Here's how the part is built. I have some questions about the finished solid (model axes, mm). Give positions to 0.01 mm unless a question says otherwise; leave off trailing zeros. Loops run counter-clockwise (first coordinate to the right, second up) from the corner with the lowest first, then second, coordinate; pieces in that order, holes last. Notation, with made-up numbers: (36, 66.5) - (46, 66.5) arc R24 cw to (46, 99.5) - close; hole circle Ø5 at (72.25, 60). An arc over 180 degrees is marked (long way). Use one line per item in the form item = value.
from build123d import *

# Parameters (mm, degrees)
F0_W     = 19.05
F0_H     = 19.05
F0_W_2   = 12.7
F1_DEPTH = 7.9375
F2_D     = 10.0838
F3_D     = 13.49248


# Not quite as in the source:
# - a feature names something its author has since deleted; it is built from what else it names


with BuildPart() as f1:
    # F0 (on Top) → F1 (new body)
    with BuildSketch(Plane.XY):
        with Locations((-66.5298237595, -51.1898304701)):
            Rectangle(F0_W, F0_H)
        Polygon((-57.0048237595, -41.6648304701), (-57.0048237595, -60.7148304701), (-37.9548237595, -60.7148304701), (-37.9548237595, 9.1351695299), (-76.0548237595, 9.1351695299), (-76.0548237595, -41.6648304701), align=None)
        Polygon((-37.9548237595, 9.1351695299), (-37.9548237595, -60.7148304701), (0.1451762405, -60.7148304701), (0.1451762405, -41.6648304701), (0.1451762405, -0.3898304701), (22.3701762405, -0.3898304701), (22.3701762405, -41.6648304701), (22.3701762405, -60.7148304701), (38.2451762405, -60.7148304701), (38.2451762405, 9.1351695299), align=None)
        Polygon((-37.9548237595, 78.9851695299), (-76.0548237595, 9.1351695299), (-37.9548237595, 9.1351695299), (-37.9548237595, 59.9351695299), align=None)
        Polygon((0.1451762405, -41.6648304701), (0.1451762405, -60.7148304701), (22.3701762405, -60.7148304701), (22.3701762405, -41.6648304701), (22.3701762405, -0.3898304701), (0.1451762405, -0.3898304701), align=None)
        Polygon((-37.9548237595, 59.9351695299), (-37.9548237595, 9.1351695299), (38.2451762405, 9.1351695299), (38.2451762405, 59.9351695299), (25.5451762405, 59.9351695299), (25.5451762405, 78.9851695299), (-25.2548237595, 78.9851695299), (-25.2548237595, 59.9351695299), align=None)
        with Locations((-31.6048237595, 69.4601695299)):
            Rectangle(F0_W_2, F0_H)
        Polygon((38.2451762405, 59.9351695299), (38.2451762405, 9.1351695299), (76.3451762405, 9.1351695299), (38.2451762405, 78.9851695299), align=None)
        Polygon((76.3451762405, 9.1351695299), (38.2451762405, 9.1351695299), (38.2451762405, -60.7148304701), (57.2951762405, -60.7148304701), (76.3451762405, -60.7148304701), align=None)
        with Locations((31.8951762405, 69.4601695299)):
            Rectangle(F0_W_2, F0_H)
    extrude(amount=F1_DEPTH)

    # F2 (through all)
    with Locations(Plane(origin=(0, 0, 0), x_dir=(1, 0, 0), z_dir=(0, 0, -1))):
        with Locations((-57.0048237595, 0.3898304701), (-57.0048237595, 41.6648304701), (0.1451762405, 0.3898304701), (0.1451762405, 41.6648304701), (57.2951762405, 0.3898304701), (57.2951762405, 41.6648304701), (-22.5665104002, 0), (-22.5665104002, 41.275), (22.3701762405, 41.6648304701), (22.3701762405, 0.3898304701)):
            Hole(F2_D / 2)

    # F3 (through all)
    with Locations(Plane(origin=(0, 0, 0), x_dir=(1, 0, 0), z_dir=(0, 0, -1))):
        with Locations((-25.2548237595, -59.9351695299), (25.5451762405, -59.9351695299)):
            Hole(F3_D / 2)


solid = f1.part
(1) For P1, Ø8, axis at x = -57, y = -41.66, coming from the -Z side; P2, Ø3, axis at y = 34, z = 7, coming from the -X side; P3, Ø3, axis at y = 27.5, z = 6, coming from the -X side, each with a flat end and sliding along its axis, tell me the tip position at first contact or that it passes through.
Geometry says:
P1 = through
P2 = -63.31
P3 = -66.86
(2) If I drill on probe 1 along Y at (x, z) = (61, 4.5); probe 2 along X at (y, z) = (-43, 4.75); probe 3 along Y at (x, z) = (-1, 6.5), over which ranges is the centre line in solid material (lowest first)?
Geometry says:
probe_1 = -60.71 to -45.08, -38.25 to -3.81, 3.03 to 37.27
probe_2 = -76.05 to -61.87, -52.14 to -27.3, -17.83 to -4.72, 5.01 to 17.51, 27.23 to 52.43, 62.16 to 76.35
probe_3 = -60.71 to -46.57, -36.75 to -5.3, 4.52 to 78.99
(3) If we section it at D-D (x = -56): List the corners of the cut face in (y, z) for me.
Geometry says:
outline = (-60.71, 0) - (-46.61, 0) - (-46.61, 7.94) - (-60.71, 7.94) - close; (-36.72, 0) - (-5.33, 0) - (-5.33, 7.94) - (-36.72, 7.94) - close; (4.55, 0) - (45.9, 0) - (45.9, 7.94) - (4.55, 7.94) - close
(4) Thinking about a two-plate mould opening in Y: for faces 1 (the flat face through (76.345, -26, 4)), 2 (the flat face through (57.562, 43.571, 3.913)), 3 (the cylindrical face through (-53.289, -45.072, 4.024)), which applies, pulls with the +Y half, pulls with the -Y half, needs draft (parallel to the pull), parting line crosses it, or undercut?
Geometry says:
face_1 = needs draft
face_2 = pulls with the +Y half
face_3 = undercut
(5) If we section it at A-A (y = 55): List the corners of the cut face in (x, z) for me.
Geometry says:
outline = (-51.04, 0) - (-29.85, 0) - (-29.85, 7.94) - (-51.04, 7.94) - close; (-20.66, 0) - (20.95, 0) - (20.95, 7.94) - (-20.66, 7.94) - close; (30.14, 0) - (51.33, 0) - (51.33, 7.94) - (30.14, 7.94) - close
(6) If we section it at B-B (x = 24): List the corners of the cut face in (y, z) for me, plus the area to 3 significant figures.
Geometry says:
outline = (-60.71, 0) - (-46.44, 0) - (-46.44, 7.94) - (-60.71, 7.94) - close; (-36.89, 0) - (-5.16, 0) - (-5.16, 7.94) - (-36.89, 7.94) - close; (4.38, 0) - (53.37, 0) - (53.37, 7.94) - (4.38, 7.94) - close; (66.5, 0) - (78.99, 0) - (78.99, 7.94) - (66.5, 7.94) - close
area = 853 mm²
(7) If we section it at C-C (z = 5): Give the number of separate pieces and of enclosed holes in the cut face, plus the area to 3 significant figures.
Geometry says:
separate_pieces = 1
enclosed_holes = 12
area = 17,500 mm²
